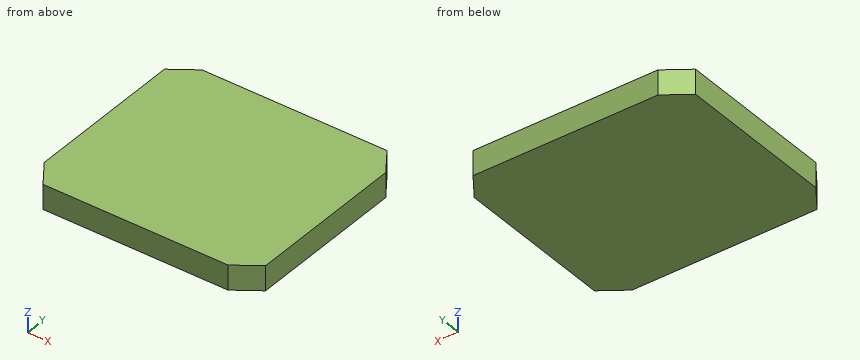
from build123d import *
from OCP.BRepFilletAPI import BRepFilletAPI_MakeChamfer

# Parameters (mm, degrees)
SKETCH_1_W      = 184
SKETCH_1_H      = 164
EXTRUDE_1_DEPTH = 20
CHAMFER_1_SIZE  = 20
CHAMFER_1_SIZE2 = 14.004150764


with BuildPart() as part:
    # 草图1 → 凸台-拉伸1 (new body)
    with BuildSketch(Plane.XY):
        Rectangle(SKETCH_1_W, SKETCH_1_H)
    extrude(amount=EXTRUDE_1_DEPTH)

    # 倒角1: one chamfer whose edges measure the first distance from different faces: ONE call of the kernel's chamfer builder (chamfer() names one face for all edges)
    chamfer_1_edges_1 = [part.edges().sort_by_distance(p)[0] for p in [
        (92, -82, 10),
    ]]
    chamfer_1_side_1 = [part.faces().sort_by_distance(p)[0] for p in [
        (0, -82, 10),
    ]]
    chamfer_1_edges_2 = [part.edges().sort_by_distance(p)[0] for p in [
        (-92, -82, 10),
    ]]
    chamfer_1_side_2 = [part.faces().sort_by_distance(p)[0] for p in [
        (-92, 0, 10),
    ]]
    chamfer_1_edges_3 = [part.edges().sort_by_distance(p)[0] for p in [
        (-92, 82, 10),
    ]]
    chamfer_1_side_3 = [part.faces().sort_by_distance(p)[0] for p in [
        (0, 82, 10),
    ]]
    chamfer_1_edges_4 = [part.edges().sort_by_distance(p)[0] for p in [
        (92, 82, 10),
    ]]
    chamfer_1_side_4 = [part.faces().sort_by_distance(p)[0] for p in [
        (92, 0, 10),
    ]]
    chamfer_1 = BRepFilletAPI_MakeChamfer(part.part.solid().wrapped)
    for e in chamfer_1_edges_1:
        chamfer_1.Add(CHAMFER_1_SIZE, CHAMFER_1_SIZE2, e.wrapped, chamfer_1_side_1[0].wrapped)  # the first distance lies on this face
    for e in chamfer_1_edges_2:
        chamfer_1.Add(CHAMFER_1_SIZE, CHAMFER_1_SIZE2, e.wrapped, chamfer_1_side_2[0].wrapped)  # the first distance lies on this face
    for e in chamfer_1_edges_3:
        chamfer_1.Add(CHAMFER_1_SIZE, CHAMFER_1_SIZE2, e.wrapped, chamfer_1_side_3[0].wrapped)  # the first distance lies on this face
    for e in chamfer_1_edges_4:
        chamfer_1.Add(CHAMFER_1_SIZE, CHAMFER_1_SIZE2, e.wrapped, chamfer_1_side_4[0].wrapped)  # the first distance lies on this face
    add(Compound.cast(chamfer_1.Shape()), mode=Mode.REPLACE)


solid = part.part
Can you work these out from the model? Positions are in its coordinate system, mm. Coordinates: 2 decimals unless noted, no trailing zeros. Order: outer loops, then holes, each group sorted by start corner. A loop starts at its lowest first (then second) coordinate and runs counter-clockwise, first axis right, second up. Notation, with made-up numbers: (-3, -3.75) - (49, -3.75) arc R27 cw to (49, 14.25) - close; hole circle Ø11 at (-2, 8.25). An arc over 180 degrees is marked (long way). Answer as a JSON object with one key per item and string values. Group by question number.
Q1. Imagine slicing it at B-B (y = -71). Please give me the cut outline in (x, z).
Q2. I need wall thicknesses on line 1 (Y direction, x = -82.5, z = 16.75); line 2 (X direction, y = 74.5, z = 3.75); line 3 (X direction, y = 68, z = 1.25). Which ranges of each line are inside material? Lowest first, please. Write a range as from..to.
Q3. Imagine slicing it at A-A (z = 14.25). Please give me the cut outline in (x, y).
Determined:
{
 "1": {"outline": "(-85.7, 0) - (87.71, 0) - (87.71, 20) - (-85.7, 20) - close"},
 "2": {"line 1": "y = -75.57..74.65", "line 2": "x = -82.71..83.25", "line 3": "x = -91.99..87.8"},
 "3": {"outline": "(-92, -62) - (-78, -82) - (72, -82) - (92, -68) - (92, 62) - (78, 82) - (-72, 82) - (-92, 68) - close"}
}
